```python
from build123d import *

# Parameters (mm, degrees)
SKETCH2_W                = 90
SKETCH2_H                = 55
BOSS_EXTRUDE1_DEPTH      = 100
SKETCH3_W                = 85
SKETCH3_H                = 50
CUT_EXTRUDE1_DEPTH       = 95
BOSS_EXTRUDE4_DEPTH      = 20
BOSS_EXTRUDE4_DEPTH_BACK = 2.5
SKETCH4_W                = 17.5
SKETCH4_H                = 30
SKETCH7_W                = 17.5
SKETCH7_H                = 2.5
CUT_EXTRUDE2_REACH       = 57
SKETCH11_W               = 10
SKETCH11_H               = 25


with BuildPart() as part:
    # Sketch2 → Boss-Extrude1 (new body)
    with BuildSketch(Plane(origin=(0, 0, 0), x_dir=(1, 0, 0), z_dir=(0, 1, 0))):
        with Locations((45, 27.5)):
            Rectangle(SKETCH2_W, SKETCH2_H)
    extrude(amount=BOSS_EXTRUDE1_DEPTH)

    # Sketch3 → Cut-Extrude1 (cut)
    with BuildSketch(Plane(origin=(0, 100, 0), x_dir=(1, 0, 0), z_dir=(0, 1, 0))):
        with Locations((45, 27.5)):
            Rectangle(SKETCH3_W, SKETCH3_H)
    extrude(amount=-CUT_EXTRUDE1_DEPTH, mode=Mode.SUBTRACT)

    # Sketch10 → Boss-Extrude4 (add, two sides)
    with BuildSketch(Plane(origin=(36.25, 0, 0), x_dir=(0, 0, -1), z_dir=(1, 0, 0))) as boss_extrude4_sk:
        Polygon((55, 30), (55, 0), (25, 0), (21.464466094, 0), (55, 33.535533906), align=None)
    extrude(amount=BOSS_EXTRUDE4_DEPTH)
    extrude(boss_extrude4_sk.sketch, amount=-BOSS_EXTRUDE4_DEPTH_BACK)

    # Sketch4 → Cut-Loft4 section 0
    with BuildSketch(Plane.XZ):
        with Locations((45, -40)):
            Rectangle(SKETCH4_W, SKETCH4_H)
    # Sketch7 → Cut-Loft4 section 1
    with BuildSketch(Plane(origin=(0, 30, 0), x_dir=(-1, 0, 0), z_dir=(0, -1, 0))):
        with Locations((-45, 53.75)):
            Rectangle(SKETCH7_W, SKETCH7_H)
    loft(mode=Mode.SUBTRACT)

    # Sketch11 → Cut-Extrude2 (cut, up to next)
    with BuildSketch(Plane.XY, mode=Mode.PRIVATE) as cut_extrude2_sk1:
        with Locations((82.5, 85)):
            Rectangle(SKETCH11_W, SKETCH11_H)
    cut_extrude2_tool1 = extrude(cut_extrude2_sk1.sketch, amount=-CUT_EXTRUDE2_REACH, mode=Mode.PRIVATE) & part.part
    add(cut_extrude2_tool1.solids().sort_by_distance((82.5, 85, 0))[0], mode=Mode.SUBTRACT)
    # Sketch11 → Cut-Extrude2 (cut, up to next)
    with BuildSketch(Plane.XY, mode=Mode.PRIVATE) as cut_extrude2_sk2:
        with Locations((7.5, 85)):
            Rectangle(SKETCH11_W, SKETCH11_H)
    cut_extrude2_tool2 = extrude(cut_extrude2_sk2.sketch, amount=-CUT_EXTRUDE2_REACH, mode=Mode.PRIVATE) & part.part
    add(cut_extrude2_tool2.solids().sort_by_distance((7.5, 85, 0))[0], mode=Mode.SUBTRACT)


solid = part.part
```
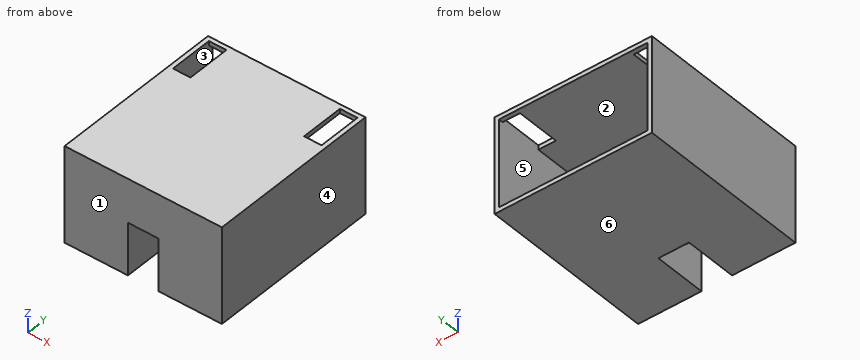
The listing builds one solid part. Answer for the finished solid, in the listing's coordinates (mm). Face numbers are marked on the shaded views. A direction names the side the tool comes from. Coordinates: 2 decimals unless noted, no trailing zeros. Write each loop counter-clockwise with the first axis right and the second up, starting at its lowest first coordinate (ties: lowest second). Pieces come first, ordered by that corner, then holes. Notation, with made-up numbers: (76.5, 86) - (100.5, 86) arc R20 cw to (100.5, 118) - close; hole circle Ø2 at (-37, 56). An arc over 180 degrees is marked (long way). One line per item, written item: value.
1) For a pull along Z with two mould halves and no side action, classify the marked faces 3, 4, 5 and 6 as pulls with the +Z half, pulls with the -Z half, needs draft (parallel to the pull), parting line crosses it, or undercut.
Geometry check:
face 3: undercut
face 4: needs draft
face 5: undercut
face 6: pulls with the -Z half
2) Consider line 1 along X through (y, z) = (94, -34); line 2 along Z through (x, y) = (60, 43); line 3 along Y through (x, z) = (23.5, -33). Determine where each line is inside the solid, lowest interval first. Write a range as from..to.
Geometry check:
line 1: x = 0..2.5, 87.5..90
line 2: z = -55..-52.5, -2.5..0
line 3: y = 0..5
3) Find section C-C (y = 36). Give the vertices of the cut face in (x, z).
Geometry check:
outline: (0, -55) - (90, -55) - (90, 0) - (0, 0) - close; hole (2.5, -52.5) - (87.5, -52.5) - (87.5, -2.5) - (2.5, -2.5) - close
4) Find section A-A (y = 91.5). Give the vertices of the cut face in (x, z), and give its area (3 significant figures).
Geometry check:
outline: (0, -55) - (90, -55) - (90, 0) - (87.5, 0) - (87.5, -52.5) - (2.5, -52.5) - (2.5, 0) - (0, 0) - close; (12.5, -2.5) - (77.5, -2.5) - (77.5, 0) - (12.5, 0) - close
area: 650 mm2
5) Find section D-D (z = -21). Give the vertices of the cut face in (x, y).
Geometry check:
outline: (0, 0) - (90, 0) - (90, 100) - (87.5, 100) - (87.5, 5) - (2.5, 5) - (2.5, 100) - (0, 100) - close
6) Each of these flat-tipped pins is pushed along its axis until it touches: pin 1 Ø6 at (x, z) = (76, -19) entering from +Y; pin 2 Ø1.2 at (x, z) = (45.5, -53) entering from -Y. Where does it stop, or does it pass through?
Geometry check:
pin 1: stops at y = 5
pin 2: stops at y = 29.89
7) A tool of negligible diameter and unlimited length cuts with its end or side. For the marked faces 1 and 2, from which of +Z, -Z, +X, -X, +Y, -Y can it reach the whole face along a straight path? Write none if from no direction.
Geometry check:
face 1: +Z, -Z, +X, -X, -Y
face 2: +Y
8) Find section B-B (x = 83.5). Give the vertices of the cut face in (y, z).
Geometry check:
outline: (0, -55) - (100, -55) - (100, -52.5) - (5, -52.5) - (5, -2.5) - (72.5, -2.5) - (72.5, 0) - (0, 0) - close; (97.5, -2.5) - (100, -2.5) - (100, 0) - (97.5, 0) - close
